Geometry check sheet. Reference: the model listing, model coordinates, mm. Face numbers are marked on the shaded views. Coordinates: 2 decimals unless noted, no trailing zeros. Write each loop counter-clockwise with the first axis right and the second up, starting at its lowest first coordinate (ties: lowest second). Pieces come first, ordered by that corner, then holes. Notation, with made-up numbers: (20, 11) -> (25, 11) arc R23 ccw to (25, 38) -> close; hole circle Ø1 at (31.5, 44). An arc over 180 degrees is marked (long way). Answer in a Markdown table with one row per item. Add a question column.
1. Cross-section at A-A on x = 31.5. Record the cut outline in (y, z).
2. Mould release check, pull along Y, two halves, no side actions. Record for the marked faces 1, 2 and 3: pulls with the +Y half, pulls with the -Y half, needs draft (parallel to the pull), parting line crosses it, or undercut.
3. Scan lines: L1, parallel to Y at x = -2.5, z = 3.75; L2, parallel to Y at x = 36, z = -1.25; L3, parallel to X at y = -3.25, z = -2.5. Record each from-to range of solid material in increasing order. Write a range as from..to.
4. Depth check by flat-ended pin: P1, Ø3, axis at x = 32.5, y = -3, coming from the +Z side; P2, Ø2, axis at x = 14, y = 2, coming from the +Z side; P3, Ø1.5, axis at x = 38.5, y = 1.5, coming from the +Z side. Enter the tip coordinate at first touch or a pass-through.
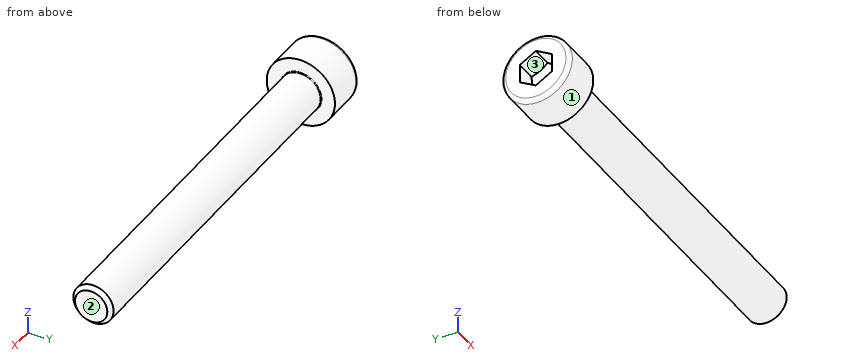
Autodesk Inventor part; units mm, degrees
ref_plane "Work Plane1" through (29, 0, 0) normal (0, -1, 0) x (1, 0, 0)
ref_plane "YZ Plane" through (0, 0, 0) normal (1, 0, 0) x (0, 1, 0)
ref_plane "XZ Plane" through (0, 0, 0) normal (0, 1, 0) x (-1, 0, 0)
sketch "Sketch1" plane through (0, 0, 0) normal (0, 0, 1) x (1, 0, 0)
  line L0 (-1.1667, 0) -> (45, 0)
  line L1 (45, 0) -> (45, 2.5)
  line L2 (45, 2.5) -> (23, 2.5)
  line L3 (23, 2.5) -> (22.5091, 2.5)
  line L4 (22.5091, 2.5) -> (0, 2.5)
  line L5 (0, 2.5) -> (0, 4.25)
  line L6 (0, 4.25) -> (-5, 4.25)
  line L7 (-5, 4.25) -> (-5, 2.3094)
  line L8 (-5, 2.3094) -> (-2.5, 2.3094)
  line L9 (-2.5, 2.3094) -> (-1.1667, 0)
  line L10 (-15, 0) -> (55, 0)
  line L11 (0, -0.85) -> (0, 5.1)
  line L12 (23, 2.5) -> (0, 2.5) construction
  dimension "d1" = 22
  dimension "d2" = 0.4909
  dimension "d3" = 5
  dimension "d4" = 2.5
  dimension "d5" = 60
  dimension "d6" = 5
  dimension "d7" = 5
  dimension "d8" = 4.6188
  dimension "d9" = 8.5
  dimension "d26" = 45
revolve "Body" add sketch "Sketch1" angle 360 about axis through (-1.1667, 0, 0) along (1, 0, 0)
sketch "Sketch2" plane through (-5, 0, 0) normal (-1, 0, 0) x (0, 0, 1)
  circle A0 centre (0, 0) radius 2.3094
  line L0 (0, -5.95) -> (0, 5.95)
  line L1 (-5.95, 0) -> (5.95, 0)
  line L2 (2.3094, 0) -> (1.1547, -2)
  line L3 (1.1547, -2) -> (-1.1547, -2)
  line L4 (-1.1547, -2) -> (-2.3094, 0)
  line L5 (-2.3094, 0) -> (-1.1547, 2)
  line L6 (-1.1547, 2) -> (1.1547, 2)
  line L7 (1.1547, 2) -> (2.3094, 0)
extrude "Slot" add sketch "Sketch2" against normal up to next contours L7 A0 | A0 L2 | L6 L0 A0 | A0 L0 L3 | L0 L6 A0 | A0 L3 L0 | L4 A0 | A0 L5
fillet "Fillet1" radius 0.5 1 edges at (-5, -4.25, 0)
thread "Thread"
chamfer "Chamfer1" distance 0.4908 distance2 0.4908 1 edges at (45, -2.5, 0) measured on face at (45, 0.4734, 0.6858)
ref_plane "Work Plane1" through (29, 0, 0) normal (0, -1, 0) x (1, 0, 0)
fillet "Fillet2" radius 0.1 1 edges at (0, -2.5, 0)
equation "\"d1\" = GEL"
equation "\"d3\" = KOH"
equation "\"d4\" = INTI"
equation "\"d6\" = GD"
equation "\"d7\" = BDM"
equation "\"d8\" = 1.1547 * SW"
equation "\"d9\" = KOD"
equation "\"d26\" = NLG"
equation "\"d30\" = R"
equation "\"d17\" = RR"
equation "\"d13\" = GEL"
equation "\"d15\" = -0.5 * SPD + 0.5 * GD"
equation "\"d16\" = GUL"
equation "\"GD\" = 5"
equation "\"NLG\" = 45"
equation "\"GEL\" = 22"
equation "\"KOD\" = 8.5"
equation "\"KOH\" = 5"
equation "\"INTI\" = 2.5"
equation "\"GAL\" = 0.61345 * PTC"
equation "\"GUL\" = 0.61345 * PTC"
equation "\"BDM\" = NND"
equation "\"SW\" = 4"
equation "\"RR\" = 0.5"
equation "\"SPD\" = NND - 1.2269 * PTC"
equation "\"R\" = 0.1"
equation "\"TOA\" = 30deg"
equation "\"GD1\" = THREADDIA - 1.2269 * PTC"
equation "\"THREADDIA\" = 5"
equation "\"FAWI\" = 45deg"
equation "\"PTC\" = 0.8"
equation "\"NND\" = 5"
equation "\"E0\" = 1.155 * SW"
properties part number "ISO 4762 - M5 x 45" material "Steel"
Results found:
| question | item | result |
|---|---|---|
| 1 | outline | circle Ø5 at (0, 0) |
| 2 | face 1 | parting line crosses it |
| 2 | face 2 | needs draft |
| 2 | face 3 | undercut |
| 3 | L1 | y = -2..2 |
| 3 | L2 | y = -2.17..2.17 |
| 3 | L3 | x = -4.86..0 |
| 4 | P1 | stops at z = 2 |
| 4 | P2 | stops at z = 2.29 |
| 4 | P3 | stops at z = 2.38 |
